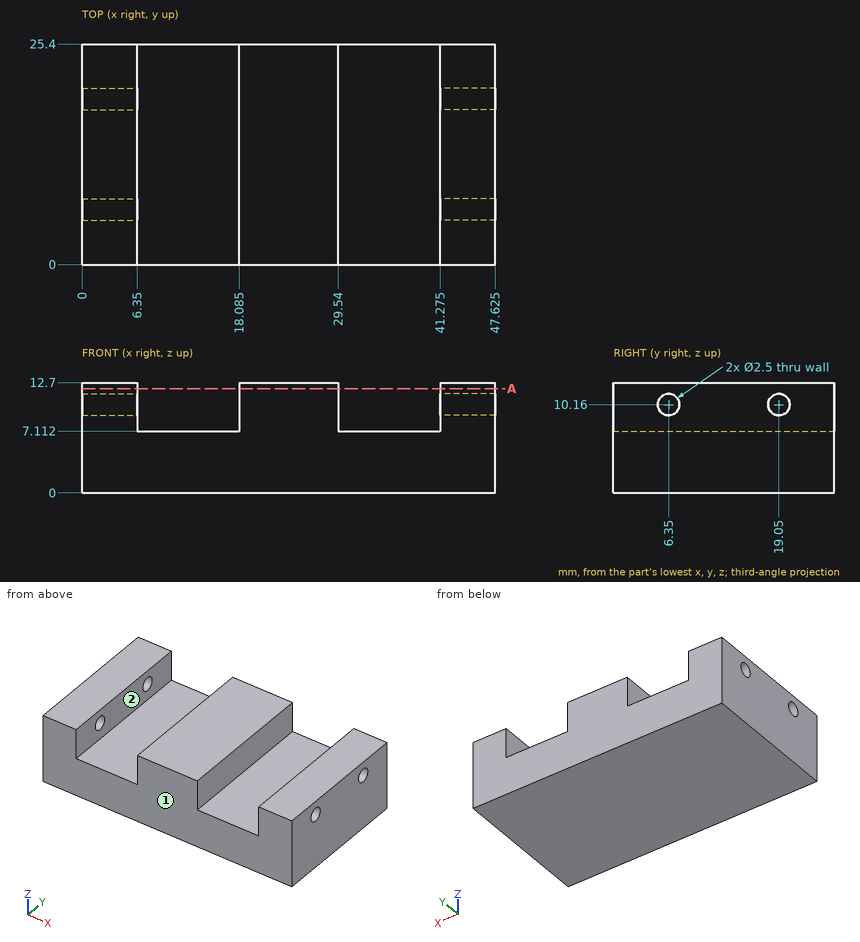
Study the drawing (mm; zero at the part's minimum x, y, z) and answer. A direction names the side the tool comes from. Coordinates: 2 decimals unless noted, no trailing zeros. Answer as a JSON object with one key per item and string values. Group by question number.
Item 1: Section A-A (z = 12) is taken. Give the number of separate pieces and of enclosed holes in the cut face.
Item 2: Consider L1, parallel to Z at x = 2, y = 6.35; L2, parallel to Z at x = 37, y = 13.5; L3, parallel to Y at x = 2, z = 10.75. Determine where each line is inside the solid, lowest interval first.
Item 3: Each of these flat-tipped pins is pushed along its axis until it touches: P1, Ø3.5, axis at x = 10, y = 9.5, coming from the +Z side; P2, Ø3, axis at y = 6.35, z = 10.16, coming from the -X side; P3, Ø2, axis at y = 19.05, z = 10.16, coming from the -X side (3 decimals); P4, Ø1.5, axis at y = 6.35, z = 10.16, coming from the +X side. Where does it stop, or does it pass through?
Item 4: Which of the six approach directions +Z, -Z, +X, -X, +Y, -Y give full straight-line access (tool end or side, diameter ignored) to the marked faces 1 and 2?
Solved:
{
 "1": {"separate pieces": "3", "enclosed holes": "0"},
 "2": {"L1": "z = 0 to 8.91, 11.41 to 12.7", "L2": "z = 0 to 7.11", "L3": "y = 0 to 5.25, 7.45 to 17.95, 20.15 to 25.4"},
 "3": {"P1": "stops at z = 7.11", "P2": "stops at x = 0", "P3": "stops at x = 18.085", "P4": "stops at x = 29.54"},
 "4": {"face 1": "+Z, -Z, +X, -X, -Y", "face 2": "+Z, +Y, -Y"}
}
